from build123d import *

# Parameters (mm, degrees)
F0_W     = 250
F0_H     = 150
F1_DEPTH = 60
F2_T     = -4
F3_W     = 38.25
F3_H     = 46
F4_DEPTH = 40
F5_W     = 80
F5_H     = 6
F6_DEPTH = 10


# Not quite as in the source:
# - a pattern or mirror of a feature is missing from the dataset's text; its kind, count and spacing are read off the source's solid


with BuildPart() as f1:
    # F0 (on Top) → F1 (new body)
    with BuildSketch(Plane.XY):
        with Locations((0.8881594986, -9.8060739803)):
            Rectangle(F0_W, F0_H)
    extrude(amount=F1_DEPTH)

    # F2
    f2_openings = [f1.faces().sort_by_distance(p)[0] for p in [
        (0.888159, -9.806074, 60),
    ]]
    offset(amount=F2_T, openings=f2_openings)

    # F3 (on face) → F4 (join)
    with BuildSketch(Plane.XY.offset(4)):
        Polygon((-81.8618405014, 15.1939260197), (-120.1118405014, 15.1939260197), (-120.1118405014, 13.1939260197), (-81.8618405014, 13.1939260197), (-81.8618405014, -32.8060739803), (-120.1118405014, -32.8060739803), (-120.1118405014, -34.8060739803), (-81.8618405014, -34.8060739803), (-81.8618405014, -80.8060739803), (-79.3618405014, -80.8060739803), (-79.3618405014, -34.8060739803), (-41.1118405014, -34.8060739803), (-41.1118405014, -80.8060739803), (-38.6118405014, -80.8060739803), (-38.6118405014, -34.8060739803), (-0.3618405014, -34.8060739803), (-0.3618405014, -80.8060739803), (2.1381594986, -80.8060739803), (2.1381594986, -34.8060739803), (40.3881594986, -34.8060739803), (40.3881594986, -80.8060739803), (42.8881594986, -80.8060739803), (42.8881594986, -34.8060739803), (81.1381594986, -34.8060739803), (81.1381594986, -80.8060739803), (83.6381594986, -80.8060739803), (83.6381594986, -34.8060739803), (121.8881594986, -34.8060739803), (121.8881594986, -32.8060739803), (83.6381594986, -32.8060739803), (83.6381594986, 13.1939260197), (121.8881594986, 13.1939260197), (121.8881594986, 15.1939260197), (83.6381594986, 15.1939260197), (83.6381594986, 61.1939260197), (81.1381594986, 61.1939260197), (81.1381594986, 15.1939260197), (42.8881594986, 15.1939260197), (42.8881594986, 61.1939260197), (40.3881594986, 61.1939260197), (40.3881594986, 15.1939260197), (2.1510550287, 15.1939260197), (2.1381594986, 15.1939260197), (2.1381594986, 61.1939260197), (-0.3618405014, 61.1939260197), (-0.3618405014, 15.1939260197), (-38.6118405014, 15.1939260197), (-38.6118405014, 61.1939260197), (-41.1118405014, 61.1939260197), (-41.1118405014, 15.1939260197), (-79.3618405014, 15.1939260197), (-79.3618405014, 61.1939260197), (-81.8618405014, 61.1939260197), align=None)
        with Locations((-60.2368405014, -9.8060739803)):
            Rectangle(F3_W, F3_H, mode=Mode.SUBTRACT)
        with Locations((-19.4868405014, -9.8060739803)):
            Rectangle(F3_W, F3_H, mode=Mode.SUBTRACT)
        with Locations((21.2631594986, -9.8060739803)):
            Rectangle(F3_W, F3_H, mode=Mode.SUBTRACT)
        with Locations((62.0131594986, -9.8060739803)):
            Rectangle(F3_W, F3_H, mode=Mode.SUBTRACT)
    extrude(amount=F4_DEPTH)

    # F5 (on face) → F6 (join)
    with BuildSketch(Plane(origin=(-124.1118405014, 0, 0), x_dir=(0, -1, 0), z_dir=(-1, 0, 0))):
        with Locations((10, 45.6811115146)):
            Rectangle(F5_W, F5_H)
    f6 = extrude(amount=F6_DEPTH)

    # F6_copies: F6 across plane
    add(f6.mirror(Plane(origin=(0, 0, 0), x_dir=(0, 0, 1), z_dir=(1, 0, 0))))


solid = f1.part
Could you check a few things on this model? Use its own coordinates, in mm. A direction names the side the tool comes from. Round coordinates to 2 decimals unless told otherwise and drop trailing zeros. Write each loop counter-clockwise with the first axis right and the second up, starting at its lowest first coordinate (ties: lowest second). Pieces come first, ordered by that corner, then holes. Notation, with made-up numbers: (44.25, 70.25) -> (102.25, 70.25) arc R25 cw to (102.25, 90.25) -> close; hole circle Ø10 at (-38, 78). An arc over 180 degrees is marked (long way). Use a Markdown table: item, result.
1. If we section it at D-D (z = 25.5): State how many separate pieces and enclosed holes the cut face has, then the cut area to 3 significant figures.
Answer key:
| item | result |
|---|---|
| separate pieces | 1 |
| enclosed holes | 18 |
| area | 5,830 mm^2 |
2. If we section it at B-B (y = -63): List the corners of the cut face in (x, z) for me.
Answer key:
| item | result |
|---|---|
| outline | (-124.11, 0) -> (125.89, 0) -> (125.89, 60) -> (121.89, 60) -> (121.89, 4) -> (83.64, 4) -> (83.64, 44) -> (81.14, 44) -> (81.14, 4) -> (42.89, 4) -> (42.89, 44) -> (40.39, 44) -> (40.39, 4) -> (2.14, 4) -> (2.14, 44) -> (-0.36, 44) -> (-0.36, 4) -> (-38.61, 4) -> (-38.61, 44) -> (-41.11, 44) -> (-41.11, 4) -> (-79.36, 4) -> (-79.36, 44) -> (-81.86, 44) -> (-81.86, 4) -> (-120.11, 4) -> (-120.11, 60) -> (-124.11, 60) -> close |
3. We'd pull the mould along X, two halves only. Please class faces 1 (the face through (130, 30, 46)), 2 (the face through (0, -9, 44)): +X half, -X half, draft (parallel to the pull), parting line (faces both ways), or undercut.
Answer key:
| item | result |
|---|---|
| face 1 | draft |
| face 2 | undercut |
4. Please list where these lines run through material, in increasing order: probe 1 along Y at (x, z) = (79.5, 30.5); probe 2 along Y at (x, z) = (-104.5, 55.5); probe 3 along X at (y, z) = (24.5, 56.5).
Answer key:
| item | result |
|---|---|
| probe 1 | y = -84.81 to -80.81, -34.81 to -32.81, 13.19 to 15.19, 61.19 to 65.19 |
| probe 2 | y = -84.81 to -80.81, 61.19 to 65.19 |
| probe 3 | x = -124.11 to -120.11, 121.89 to 125.89 |
5. Which directions (+Z, -Z, +X, -X, +Y, -Y) give clear straight access to the entire face, cutting with the end or side of a thin tool? Please do faces 3 (the face through (130, -9, 48.681)), 4 (the face through (-1, -84.806, 30)), 5 (the face through (-129, 30, 46)), 6 (the face through (-20, -34.806, 24)).
Answer key:
| item | result |
|---|---|
| face 3 | +Z, +X, +Y, -Y |
| face 4 | +Z, -Z, +X, -X, -Y |
| face 5 | +Z, -Z, -X, +Y |
| face 6 | +Z |
6. If we section it at C-C (x = 96): List the corners of the cut face in (y, z) for me.
Answer key:
| item | result |
|---|---|
| outline | (-84.81, 0) -> (65.19, 0) -> (65.19, 60) -> (61.19, 60) -> (61.19, 4) -> (15.19, 4) -> (15.19, 44) -> (13.19, 44) -> (13.19, 4) -> (-32.81, 4) -> (-32.81, 44) -> (-34.81, 44) -> (-34.81, 4) -> (-80.81, 4) -> (-80.81, 60) -> (-84.81, 60) -> close |
7. If we section it at A-A (z = 53): List the corners of the cut face in (x, y) for me.
Answer key:
| item | result |
|---|---|
| outline | (-124.11, -84.81) -> (125.89, -84.81) -> (125.89, 65.19) -> (-124.11, 65.19) -> close; hole (-120.11, -80.81) -> (121.89, -80.81) -> (121.89, 61.19) -> (-120.11, 61.19) -> close |
8. For pin 1 Ø12 at (y, z) = (-17, 21) entering from +X; pin 2 Ø12 at (y, z) = (-50, 27.5) entering from -X; pin 3 Ø2 at (x, y) = (-11.5, 7.5) entering from +Z, each with a flat end and sliding along its axis, tell me the tip position at first contact or that it passes through.
Answer key:
| item | result |
|---|---|
| pin 1 | stops at x = 125.89 |
| pin 2 | stops at x = -124.11 |
| pin 3 | stops at z = 4 |
